Solid Edge part; units mm, degrees
sketch "Sketch1" plane through (0, 0, 0) normal (0, 0, 1) x (1, 0, 0)
  line L0 (44.556, 10.0434) -> (100.0609, 42.0892)
  line L1 (27.5, 18.6713) -> (92.0609, 55.9456)
  line L2 (27.5, 18.6713) -> (27.5, -29.8921)
  line L3 (93.5003, -134.0471) -> (27.5, -29.8921)
  line L4 (38.0069, -16.5809) -> (107.0154, -125.483)
  arc A0 (38.0069, -16.5809) -> (44.556, 10.0434) centre (54.056, -6.4111) cw
  arc A1 (92.0609, 55.9456) -> (100.0609, 42.0892) centre (107.0495, 55.3617) cw
  arc A2 (107.0154, -125.483) -> (93.5003, -134.0471) centre (107.0495, -140.483) cw
  circle A3 centre (107.0495, 49.7048) radius 1
  circle A4 centre (101.3927, 55.3617) radius 1
  circle A5 centre (107.0495, 61.0185) radius 1
  circle A6 centre (112.7064, 55.3617) radius 1
  circle A7 centre (101.3927, -140.483) radius 1
  circle A8 centre (107.0495, -134.8261) radius 1
  circle A9 centre (112.7064, -140.483) radius 1
  circle A10 centre (107.0495, -146.1398) radius 1
extrude "Protrusion1" add sketch "Sketch1" along normal blind 5.5
Verification items for the finished model (mm, model axes). A direction names the side the tool comes from. Give positions to 0.01 mm unless a question says otherwise; leave off trailing zeros. Order: outer loops, then holes, each group sorted by start corner. A loop starts at its lowest first (then second) coordinate and runs counter-clockwise, first axis right, second up. Notation, with made-up numbers: M 11.25,24 L 70.25,24 A18 ccw 70.25,34 Z; hole C 6,-17 d1. An arc over 180 degrees is marked long. Answer in a Markdown table with one row per item. Add a question column.
Item 1: Section check C-C, the plane y = -36.5. Enter the section's corners in (x, z), and give its area (3 significant figures).
Item 2: Scan lines: probe 1 along Y at (x, z) = (91, 2.75); probe 2 along Y at (x, z) = (62, 4.95); probe 3 along X at (y, z) = (-135, 1.3). Record each from-to range of solid material in increasing order. Write a range as from..to.
Item 3: Mould release check, pull along Y, two halves, no side actions. Record for faces 3 (the cylindrical face through (115.53, -152.855, 2.712)), 4 (the flat face through (59.33, 37.05, 2.71)), 5 (the flat face through (27.5, -5, 3)): released by +Y, released by -Y, zero draft, split by the parting line, or undercut.
Item 4: Gauge pin test, flat ends, axial feed: pin 1 (2 mm diameter, centred on y = -58.5, z = 5, fed in from +X); pin 2 (1 mm diameter, centred on x = 82, y = -96.5, fed in from -Z); pin 3 (3 mm diameter, centred on x = 101, z = 3, fed in from +Y); pin 4 (1.6 mm diameter, centred on x = 107.05, y = 49.7, fed in from -Z). Record the tip position at first contact, or that the pin passes through.
Item 5: Section check A-A, the plane x = 82. Enter the section's corners in (y, z), and give its area (3 significant figures).
Item 6: Section check B-B, the plane z = 3.25. State how many separate pieces and enclosed holes the cut face has, and give its area (3 significant figures).
Item 7: Tool access check on faces 1 (the flat face through (47, -34, 0)), 2 (the flat face through (72.03, -70.27, 2.71)). Record the directions out of +Z, -Z, +X, -X, +Y, -Y that give a thin tool (end or side, any length) a straight path to the whole face; none if there is none.
Filled sheet:
| question | item | result |
|---|---|---|
| 1 | outline | M 31.69,0 L 50.63,0 L 50.63,5.5 L 31.69,5.5 Z |
| 1 | area | 104 mm^2 |
| 2 | probe 1 | y = -130.1..-100.21, 36.86..55.33 |
| 2 | probe 2 | y = -84.34..-54.44, 20.11..38.59 |
| 2 | probe 3 | x = 93.09..106.06, 108.03..121.01 |
| 3 | face 3 | undercut |
| 3 | face 4 | released by +Y |
| 3 | face 5 | zero draft |
| 4 | pin 1 | stops at x = 65.2 |
| 4 | pin 2 | stops at z = 0 |
| 4 | pin 3 | stops at y = 69.66 |
| 4 | pin 4 | passes through |
| 5 | outline | M -115.9,0 L -86.01,0 L -86.01,5.5 L -115.9,5.5 Z; M 31.66,0 L 50.14,0 L 50.14,5.5 L 31.66,5.5 Z |
| 5 | area | 266 mm^2 |
| 6 | separate pieces | 1 |
| 6 | enclosed holes | 8 |
| 6 | area | 4,870 mm^2 |
| 7 | face 1 | -Z, +X, -X, +Y, -Y |
| 7 | face 2 | +Z, -Z, +X |
